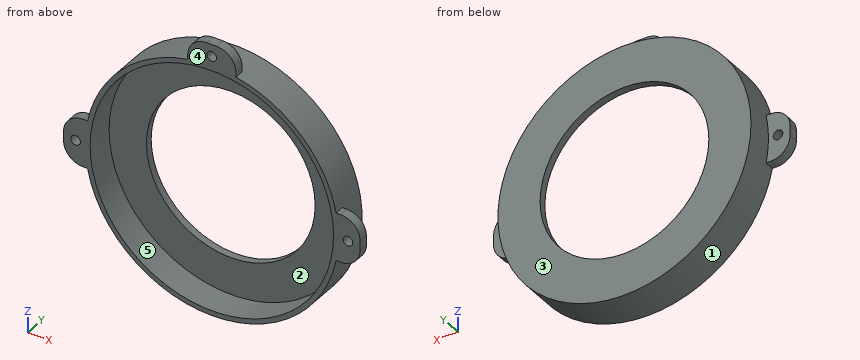
Autodesk Inventor part; units mm, degrees
ref_plane "YZ Plane" through (0, 0, 0) normal (1, 0, 0) x (0, 1, 0)
ref_plane "XZ Plane" through (0, 0, 0) normal (0, 1, 0) x (-1, 0, 0)
ref_plane "XY Plane" through (0, 0, 0) normal (0, 0, 1) x (1, 0, 0)
sketch "Sketch1" plane through (0, 0, 0) normal (0, 1, 0) x (-1, 0, 0)
  circle A0 centre (0, 0) radius 25.25
  circle A1 centre (0, 0) radius 26.25
  dimension "d0" = 50.5
  dimension "d1" = 52.5
extrude "Extrusion1" add sketch "Sketch1" along normal blind 7.5
sketch "Sketch2" plane through (0, 7.5, 0) normal (0, 1, 0) x (1, 0, 0)
  circle A0 centre (0, 0) radius 25.25
  circle A1 centre (0, 0) radius 25.25
  circle A2 centre (0, 0) radius 26.25
  circle A3 centre (0, 0) radius 17.5
  dimension "d4" = 35
extrude "Extrusion2" add sketch "Sketch2" against normal blind 1.5 contours A0
sketch "Sketch3" plane through (0, 0, 0) normal (0, -1, 0) x (1, 0, 0)
  circle A0 centre (0, 0) radius 26.25
  circle A1 centre (0, 0) radius 26.25
  line L0 (26.25, -0.0057) -> (25.75, -0.0057)
  line L1 (-26.25, 0.0058) -> (-25.75, 0.0058)
  line L2 (-0.0095, 26.25) -> (-0.0095, 25.75)
  line L3 (25.75, -0.0057) -> (25.7683, -5.0057)
  line L4 (25.7683, -5.0057) -> (30.7683, -4.9874)
  line L5 (30.7683, -4.9874) -> (30.7317, 5.0125)
  line L6 (30.7317, 5.0125) -> (25.7317, 4.9942)
  line L7 (25.7317, 4.9942) -> (25.7317, 4.9942)
  line L8 (25.75, -0.0057) -> (25.7317, 4.9942)
  line L9 (-0.0095, 25.75) -> (-5.0095, 25.75)
  line L10 (-0.0095, 25.75) -> (4.9905, 25.75) construction
  line L11 (-5.0095, 25.75) -> (-5.0095, 30.75)
  line L12 (-5.0095, 30.75) -> (4.9905, 30.75)
  line L13 (4.9905, 30.75) -> (4.9905, 25.75)
  line L14 (4.9905, 25.75) -> (-0.0095, 25.75)
  line L15 (-25.75, 0.0058) -> (-25.75, -4.9942)
  line L16 (-25.75, 0.0058) -> (-20.75, 0.0058) construction
  line L17 (-25.75, -4.9942) -> (-30.75, -4.9942)
  line L18 (-30.75, -4.9942) -> (-30.75, 5.0058)
  line L19 (-30.75, 5.0058) -> (-25.75, 5.0058)
  line L20 (-25.75, 5.0058) -> (-25.75, 0.0058)
  circle A2 centre (28.2317, 0.0058) radius 1
  circle A3 centre (-28.25, 0.0058) radius 1
  circle A4 centre (-0.0095, 28.25) radius 1
  dimension "d7" = 0.5
  dimension "d8" = 0.5
  dimension "d9" = 0.5
  dimension "d10" = 5
  dimension "d11" = 5
  dimension "d12" = 10
  dimension "d13" = 5
  dimension "d14" = 180
  dimension "d15" = 5
  dimension "d16" = 10
  dimension "d17" = 5
  dimension "d18" = 90
  dimension "d19" = 5
  dimension "d20" = 90
  dimension "d21" = 5
  dimension "d22" = 10
  dimension "d23" = 90
  dimension "d24" = 2
  dimension "d25" = 2
  dimension "d26" = 2
extrude "Extrusion3" add sketch "Sketch3" against normal blind 2 contours A0 L6 L5 L4 | L0 L8 L6 A0 | L17 L18 L19 A0 | A0 L1 L15 L17 | A0 L19 L20 L1 | L13 L14 L2 A0 | A0 L11 L12 L13 | A0 L2 L9 L11
fillet "Fillet1" radius 4 6 edges at (-30.75, 1, -4.9942) (-30.75, 1, 5.0058) (-5.0095, 1, 30.75) (4.9905, 1, 30.75) (30.7317, 1, 5.0125) (30.7683, 1, -4.9874)
properties part number "AudioColor"
Source: CAD feature listing. Evaluate the final solid. Frame: model axes, mm. Face numbers are marked on the shaded views. A direction names the side the tool comes from. Coordinates: 2 decimals unless noted, no trailing zeros. Loops run counter-clockwise (first coordinate to the right, second up) from the corner with the lowest first, then second, coordinate; pieces in that order, holes last. Notation, with made-up numbers: (86, -30.75) - (123, -30.75) arc R25 ccw to (123, -12.75) - close; hole circle Ø7 at (1, -13.75). An arc over 180 degrees is marked (long way). One line per question, with ' | ' between items.
1) Line query: line 1 along Y through (x, z) = (-16, -11); line 2 along Z through (x, y) = (12, 2); line 3 along Z through (x, y) = (18.5, 4.5). Output: solid intervals per line, ascending.
Report:
line 1: y = 6 to 7.5 | line 2: z = -23.35 to -22.22, 22.22 to 23.35 | line 3: z = -18.62 to -17.18, 17.18 to 18.62
2) Section C-C, the plane y = 1.25. Return loops of the section in (x, z).
Report:
outline: (-30.75, -0.99) arc R4 ccw to (-26.75, -4.99) - (-25.77, -4.99) arc R26.25 ccw to (25.77, -5.01) - (26.77, -5) arc R4 ccw to (30.75, -0.99) - (30.75, 1.01) arc R4 ccw to (26.73, 5) - (25.77, 4.99) arc R26.25 ccw to (4.99, 25.77) - (4.99, 26.75) arc R4 ccw to (0.99, 30.75) - (-1.01, 30.75) arc R4 ccw to (-5.01, 26.75) - (-5.01, 25.77) arc R26.25 ccw to (-25.77, 5.01) - (-26.75, 5.01) arc R4 ccw to (-30.75, 1.01) - close; hole circle Ø2 at (-28.25, 0.01); hole circle Ø50.5 at (0, 0); hole circle Ø2 at (-0.01, 28.25); hole circle Ø2 at (28.23, 0.01)
3) Section A-A, the plane x = -6. Return loops of the section in (y, z), then the cut area to 3 significant figures.
Report:
outline: (0, -25.56) - (7.5, -25.56) - (7.5, -16.44) - (6, -16.44) - (6, -24.53) - (0, -24.53) - close; (0, 24.53) - (6, 24.53) - (6, 16.44) - (7.5, 16.44) - (7.5, 25.56) - (0, 25.56) - close | area: 39.7 mm²
4) Section D-D, the plane y = 4.5. Return loops of the section in (x, z), then the cut area to 3 significant figures.
Report:
outline: circle Ø52.5 at (0, 0); hole circle Ø50.5 at (0, 0) | area: 162 mm²
5) First-contact query: P1, Ø4, axis at x = -28, z = 0.5, coming from the +Y side; P2, Ø3, axis at x = 16, y = 4.5, coming from the -Z side; P3, Ø1.5, axis at y = 3.5, z = 17, coming from the -X side; P4, Ø1.5, axis at y = 3.5, z = 9.5, coming from the +X side. Flat tips, straight axial feed; report the tip coordinate or a pass-through.
Report:
P1: stops at y = 7.5 | P2: stops at z = -21.88 | P3: stops at x = -20.62 | P4: stops at x = 24.75
6) Pull-direction query (Z, two-part tool) for the marked faces 1, 2 and 3; classes: released by +Z, released by -Z, zero draft, split by the parting line, or undercut.
Report:
face 1: split by the parting line | face 2: undercut | face 3: zero draft
7) Section B-B, the plane z = 16.5. Return loops of the section in (x, y).
Report:
outline: (-20.42, 0) - (-19.11, 0) - (-19.11, 6) - (-5.83, 6) - (-5.83, 7.5) - (-20.42, 7.5) - close; (5.83, 6) - (19.11, 6) - (19.11, 0) - (20.42, 0) - (20.42, 7.5) - (5.83, 7.5) - close
8) Set-up query: the marked faces 4 and 5. Return all of +Z, -Z, +X, -X, +Y, -Y with unobstructed straight access to the full face (end or side cutting, diameter ignored); none if empty.
Report:
face 4: +Z, -Z, +X, -X, -Y | face 5: -Y
